```python
from build123d import *

# Parameters (mm, degrees)
F0_W       = 41.4983332157
F0_H       = 50.7746972144
F0_R       = 9.7686704189
F1_DEPTH   = 62.484
F2_R       = 15.6433873562
F1_FACE1_W = 41.4983332157
F1_FACE1_H = 50.7746972144
F1_FACE1_R = 9.7686704189
F3_DEPTH   = 108.966
F4_R       = 17.7535536274
F5_DEPTH   = 148.844


with BuildPart() as f1:
    # F0 (on Front) → F1 (new body)
    with BuildSketch(Plane.XZ):
        with Locations((-87.555155158, -25.3873486072)):
            Rectangle(F0_W, F0_H)
        with Locations((-91.3773775101, -25.3873486072)):
            Circle(F0_R, mode=Mode.SUBTRACT)
    extrude(amount=-F1_DEPTH)

    # F2 (on face) + F1_face1 (on face) → F3 (join)
    with BuildSketch(Plane.XZ):
        with Locations((-91.3773775101, -25.3873486072)):
            Circle(F2_R)
    with BuildSketch(Plane(origin=(-86.9211204596, 62.484, -25.3873486072), x_dir=(1, 0, 0), z_dir=(0, 1, 0))):
        with Locations((-0.6340346985, 0)):
            Rectangle(F1_FACE1_W, F1_FACE1_H)
        with Locations((-4.4562570505, 0)):
            Circle(F1_FACE1_R, mode=Mode.SUBTRACT)
    extrude(amount=F3_DEPTH, dir=(0, -1, 0))

    # F4 (on face) → F5 (join)
    with BuildSketch(Plane(origin=(0, 62.484, 0), x_dir=(-1, 0, 0), z_dir=(0, 1, 0))):
        with Locations((91.3773775101, -25.3873486072)):
            Circle(F4_R)
    extrude(amount=F5_DEPTH)


solid = f1.part
```
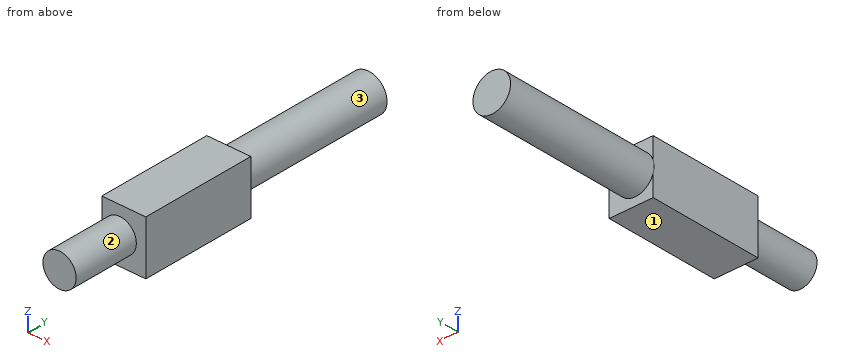
Design review of the part built by this model. Coordinates are the model's own, in mm. Face numbers are marked on the shaded views. A direction names the side the tool comes from. Coordinates: 2 decimals unless noted, no trailing zeros. Write each loop counter-clockwise with the first axis right and the second up, starting at its lowest first coordinate (ties: lowest second). Pieces come first, ordered by that corner, then holes. Notation, with made-up numbers: M 15.25,-30 L 41.25,-30 A16 cw 41.25,-13 Z; hole C 89.25,-12.5 d11. An arc over 180 degrees is marked long. Answer as a JSON object with one key per item and string values.
Item 1: Add section B-B, the plane z = -38. Give the boundary of the cut face in (x, y), and give its area (3 significant figures).
Outcome:
{"outline": "M -108.3,-46.48 L -100.63,-46.48 L -100.63,-108.97 L -82.12,-108.97 L -82.12,-46.48 L -66.81,-46.48 L -66.81,62.48 L -78.88,62.48 L -78.88,211.33 L -103.87,211.33 L -103.87,62.48 L -108.3,62.48 Z", "area": "9,400 mm²"}
Item 2: Insertion check: pin 1 Ø1.5 at (y, z) = (52, -6) entering from -X; pin 2 Ø2 at (y, z) = (169.5, -18.5) entering from +X; pin 3 Ø2 at (x, z) = (-91, -5) entering from -Y. Each pin has a flat end and moves straight along its axis. Give the tip position at first contact, or say it passes through.
Outcome:
{"pin 1": "x = -108.3", "pin 2": "x = -74.63", "pin 3": "y = -46.48"}
Item 3: Add section C-C, the plane y = 40.5. Give the boundary of the cut face in (x, z).
Outcome:
{"outline": "M -108.3,-50.77 L -66.81,-50.77 L -66.81,0 L -108.3,0 Z; hole C -91.38,-25.39 d19.54"}
Item 4: Machinability: for the marked faces 1, 2 and 3, which of the approach directions +Z, -Z, +X, -X, +Y, -Y give a long, thin tool a straight path to every point of the face, cutting with its end or side? Answer none if there is none.
Outcome:
{"face 1": "-Z, +X, -X, +Y, -Y", "face 2": "-Y", "face 3": "+Y"}
Item 5: Add section D-D, the plane y = -17. Give the boundary of the cut face in (x, z), and give its area (3 significant figures).
Outcome:
{"outline": "M -108.3,-50.77 L -66.81,-50.77 L -66.81,0 L -108.3,0 Z", "area": "2,110 mm²"}
Item 6: Add section A-A, the plane x = -95.5. Give the boundary of the cut face in (y, z), and give its area (3 significant figures).
Outcome:
{"outline": "M -108.97,-40.48 L -46.48,-40.48 L -46.48,-50.77 L 62.48,-50.77 L 62.48,-42.66 L 211.33,-42.66 L 211.33,-8.12 L 62.48,-8.12 L 62.48,0 L -46.48,0 L -46.48,-10.3 L -108.97,-10.3 Z; hole M 0,-34.24 L 62.48,-34.24 L 62.48,-16.53 L 0,-16.53 Z", "area": "11,500 mm²"}
Item 7: Wall thickness on probe 1 along Y at (x, z) = (-91, -24); probe 2 along Z at (x, y) = (-92.5, 43.5); probe 3 along Y at (x, z) = (-70.5, -47): over which ranges is each line inside the solid? List them lowest first.
Outcome:
{"probe 1": "-108.97 to 0, 62.48 to 211.33", "probe 2": "-50.77 to -35.09, -15.68 to 0", "probe 3": "-46.48 to 62.48"}
